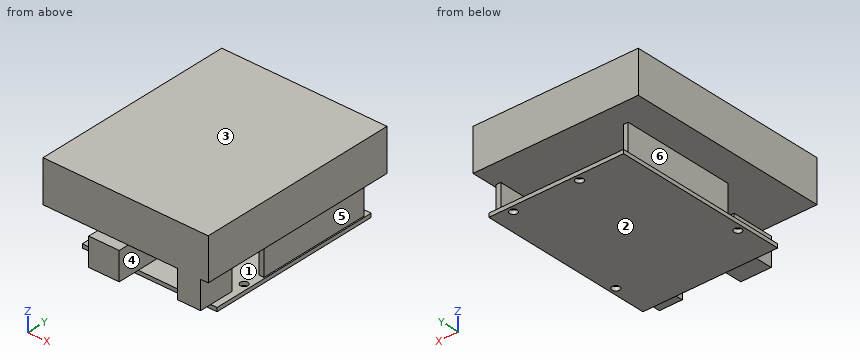
Autodesk Inventor part; units mm, degrees
ref_plane "YZ Plane" through (0, 0, 0) normal (1, 0, 0) x (0, 1, 0)
ref_plane "XZ Plane" through (0, 0, 0) normal (0, 1, 0) x (-1, 0, 0)
ref_plane "XY Plane" through (0, 0, 0) normal (0, 0, 1) x (1, 0, 0)
sketch "스케치2" plane through (0, 0, 0) normal (0, 0, 1) x (1, 0, 0)
  line L0 (-26.5, -34.5) -> (26.5, -34.5)
  line L1 (26.5, -34.5) -> (26.5, 34.5)
  line L2 (26.5, 34.5) -> (-26.5, 34.5)
  line L3 (-26.5, 34.5) -> (-26.5, -34.5)
  line L4 (-26.5, -34.5) -> (26.5, 34.5) construction
  line L5 (26.5, -34.5) -> (-26.5, 34.5) construction
  circle A0 centre (19, 32) radius 1.5
  circle A1 centre (-7, 32) radius 1.5
  circle A2 centre (24, -19.5) radius 1.5
  circle A3 centre (-24, -19.5) radius 1.5
  point P0 (0, 0)
  dimension "d0" = 53
  dimension "d1" = 69
  dimension "d2" = 3
  dimension "d3" = 3
  dimension "d4" = 2.5
  dimension "d5" = 2.5
  dimension "d6" = 7.5
  dimension "d8" = 26
  dimension "d9" = 3
  dimension "d10" = 3
  dimension "d11" = 2.5
  dimension "d12" = 2.5
  dimension "d13" = 15
extrude "돌출1" add sketch "스케치2" along normal blind 1.5
sketch "스케치3" plane through (0, 0, 1.5) normal (0, 0, 1) x (1, 0, 0)
  line L0 (-16.5, -26.3) -> (-4.5, -26.3)
  line L1 (-4.5, -26.3) -> (-4.5, -43)
  line L2 (-4.5, -43) -> (-16.5, -43)
  line L3 (-16.5, -43) -> (-16.5, -26.3)
  line L4 (-16.5, -26.3) -> (-4.5, -43) construction
  line L5 (-4.5, -26.3) -> (-16.5, -43) construction
  line L6 (15, -25) -> (24, -25)
  line L7 (24, -25) -> (24, -39)
  line L8 (24, -39) -> (15, -39)
  line L9 (15, -39) -> (15, -25)
  line L10 (15, -25) -> (24, -39) construction
  line L11 (24, -25) -> (15, -39) construction
  line L12 (-26.5, -34.5) -> (26.5, -34.5)
  line L13 (26.5, -34.5) -> (26.5, 34.5)
  line L14 (-26.5, 34.5) -> (-26.5, -34.5)
  point P0 (0, 0)
  point P1 (-10.5, -34.65)
  point P2 (19.5, -32)
  dimension "d16" = 12
  dimension "d17" = 16.7
  dimension "d18" = 9
  dimension "d19" = 14
  dimension "d20" = 4.5
  dimension "d21" = 2.5
  dimension "d22" = 8.5
  dimension "d23" = 10
extrude "돌출2" add sketch "스케치3" along normal blind 11 contours L0 L1 L12 L3 | L12 L1 L2 L3
extrude "돌출3" add sketch "스케치3" along normal blind 11 contours L9 L6 L7 L12 | L12 L7 L8 L9
sketch "스케치4" plane through (0, 0, 1.5) normal (0, 0, 1) x (1, 0, 0)
  line L0 (-25.9905, -12.9426) -> (-24.0965, -12.9426)
  line L1 (-24.0965, -12.9426) -> (-24.0965, 31.8831)
  line L2 (-24.0965, 31.8831) -> (-25.9905, 31.8831)
  line L3 (-25.9905, 31.8831) -> (-25.9905, -12.9426)
  line L4 (-25.9905, -12.9426) -> (-24.0965, 31.8831) construction
  line L5 (-24.0965, -12.9426) -> (-25.9905, 31.8831) construction
  line L6 (0, 0) -> (0, 9.4702)
  line L7 (25.9905, -12.9426) -> (24.0965, -12.9426)
  line L8 (24.0965, -12.9426) -> (24.0965, 31.8831)
  line L9 (24.0965, 31.8831) -> (25.9905, 31.8831)
  line L10 (25.9905, 31.8831) -> (25.9905, -12.9426)
  line L11 (25.9905, -12.9426) -> (24.0965, 31.8831) construction
  line L12 (24.0965, -12.9426) -> (25.9905, 31.8831) construction
  point P0 (-25.0435, 9.4702)
  point P1 (25.0435, 9.4702)
extrude "돌출4" add sketch "스케치4" along normal blind 11
sketch "스케치5" plane through (0, 0, 12.5) normal (0, 0, 1) x (1, 0, 0)
  line L0 (-38, -39) -> (27, -39)
  line L1 (27, -39) -> (27, 41)
  line L2 (27, 41) -> (-38, 41)
  line L3 (-38, 41) -> (-38, -39)
  line L4 (-38, -39) -> (27, 41) construction
  line L5 (27, -39) -> (-38, 41) construction
  line L6 (26.5, -34.5) -> (26.5, 34.5)
  point P0 (0, 0)
  point P1 (-5.5, 1)
  point P2 (-38, 34.5)
  point P3 (24, -39)
  dimension "d30" = 80
  dimension "d31" = 65
  dimension "d34" = 0.5
extrude "돌출5" add sketch "스케치5" along normal blind 16.5
properties part number "스피커"
Input: part model. Units: mm. Frame: model coordinates. Face numbers are marked on the shaded views. A direction names the side the tool comes from. Coordinates: 2 decimals unless noted, no trailing zeros. Loops run counter-clockwise (first coordinate to the right, second up) from the corner with the lowest first, then second, coordinate; pieces in that order, holes last. Notation, with made-up numbers: (-3.5, 13.5) -> (43.5, 13.5) arc R12 ccw to (43.5, 22.5) -> close; hole circle Ø8 at (57, -10). An arc over 180 degrees is marked (long way). One line per item, written item: value.
(1) Set-up query: the marked faces 4, 5 and 6. Return all of +Z, -Z, +X, -X, +Y, -Y with unobstructed straight access to the full face (end or side cutting, diameter ignored); none if empty.
Answer below:
face 4: +Y, -Y
face 5: +X, +Y, -Y
face 6: -X, +Y, -Y
(2) Pin query (flat end, axial travel): pin 1 Ø2 at (x, y) = (20, -38) entering from -Z; pin 2 Ø5.5 at (y, z) = (18, 5) entering from -X; pin 3 Ø0.8 at (x, z) = (10.5, 0.5) entering from +Y; pin 4 Ø3 at (y, z) = (-15.5, 10) entering from +X. Return the tip coordinate at first contact, or that it passes through.
Answer below:
pin 1: stops at z = 1.5
pin 2: stops at x = -25.99
pin 3: stops at y = 34.5
pin 4: passes through
(3) Cut plane A-A (y = 12). Output: boundary loops of the cut face in (x, z), then the cut area to 3 significant figures.
Answer below:
outline: (-38, 12.5) -> (-25.99, 12.5) -> (-25.99, 1.5) -> (-26.5, 1.5) -> (-26.5, 0) -> (26.5, 0) -> (26.5, 1.5) -> (25.99, 1.5) -> (25.99, 12.5) -> (27, 12.5) -> (27, 29) -> (-38, 29) -> close; hole (-24.1, 1.5) -> (24.1, 1.5) -> (24.1, 12.5) -> (-24.1, 12.5) -> close
area: 1,190 mm2
(4) Draft query along Z for the marked faces 1, 2 and 3. Return one class per face: pulls with the +Z half, pulls with the -Z half, needs draft (parallel to the pull), parting line crosses it, or undercut.
Answer below:
face 1: undercut
face 2: pulls with the -Z half
face 3: pulls with the +Z half
(5) Cut plane C-C (z = 11). Output: boundary loops of the cut face in (x, y).
Answer below:
outline: (-25.99, -12.94) -> (-24.1, -12.94) -> (-24.1, 31.88) -> (-25.99, 31.88) -> close; (-16.5, -43) -> (-4.5, -43) -> (-4.5, -26.3) -> (-16.5, -26.3) -> close; (15, -39) -> (24, -39) -> (24, -25) -> (15, -25) -> close; (24.1, -12.94) -> (25.99, -12.94) -> (25.99, 31.88) -> (24.1, 31.88) -> close
(6) Cut plane D-D (x = -15). Output: boundary loops of the cut face in (y, z), then the cut area to 3 significant figures.
Answer below:
outline: (-43, 1.5) -> (-34.5, 1.5) -> (-34.5, 0) -> (34.5, 0) -> (34.5, 1.5) -> (-26.3, 1.5) -> (-26.3, 12.5) -> (41, 12.5) -> (41, 29) -> (-39, 29) -> (-39, 12.5) -> (-43, 12.5) -> close
area: 1,610 mm2
(7) Cut plane B-B (x = 19). Output: boundary loops of the cut face in (y, z), then the cut area to 3 significant figures.
Answer below:
outline: (-39, 1.5) -> (-34.5, 1.5) -> (-34.5, 0) -> (30.5, 0) -> (30.5, 1.5) -> (-25, 1.5) -> (-25, 12.5) -> (41, 12.5) -> (41, 29) -> (-39, 29) -> close; (33.5, 0) -> (34.5, 0) -> (34.5, 1.5) -> (33.5, 1.5) -> close
area: 1,570 mm2
(8) Ray query, line 1 along Y through (x, z) = (19, 0.8); line 2 along Z through (x, y) = (11, -21); line 3 along Y through (x, z) = (-24, 1). Return the intervals inside material, ascending.
Answer below:
line 1: y = -34.5 to 30.5, 33.5 to 34.5
line 2: z = 0 to 1.5, 12.5 to 29
line 3: y = -34.5 to -21, -18 to 34.5
